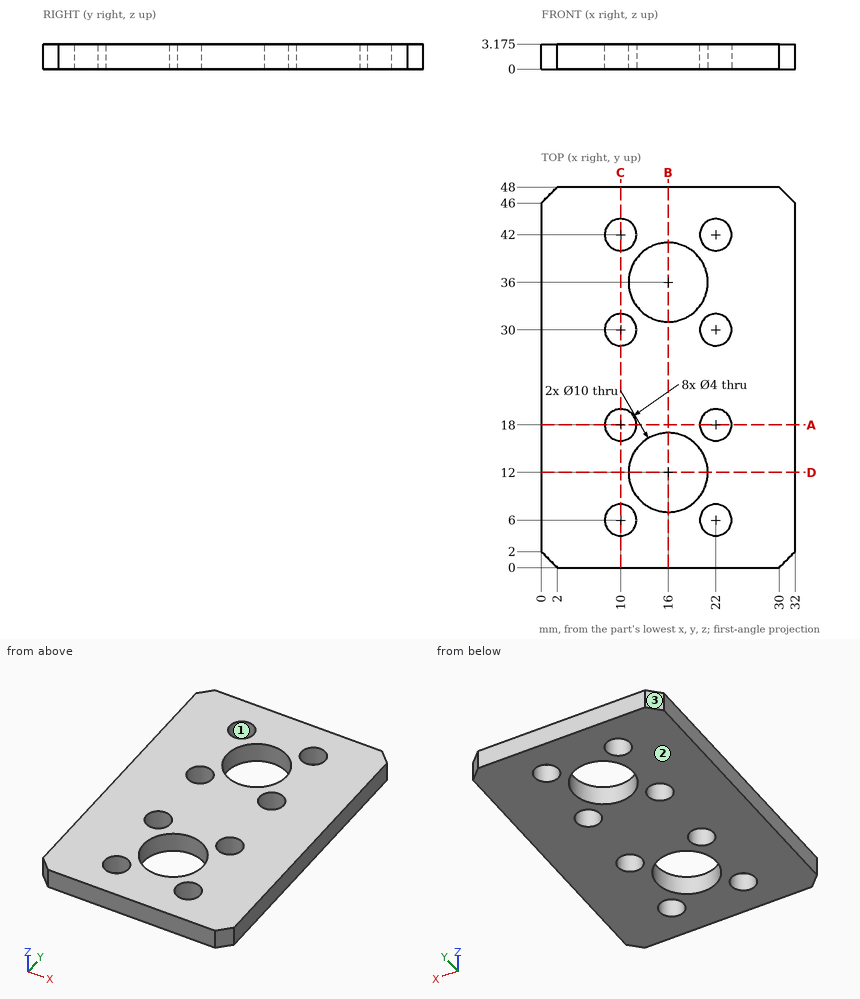
For this review, use the dimensioned drawing (mm, ordinates from the lowest corner) and the shaded views. Give positions to 0.01 mm unless a question says otherwise; leave off trailing zeros. Write each loop counter-clockwise with the first axis right and the second up, starting at its lowest first coordinate (ties: lowest second). Pieces come first, ordered by that corner, then holes. Notation, with made-up numbers: M 63,-9.75 L 98,-9.75 A11 cw 98,7.25 Z; hole C -8,22.5 d6. An arc over 180 degrees is marked long. Answer as a JSON object with one key per item and string values. Group by question number.
1) For line 1 along Y through (x, z) = (16, 0.75); line 2 along Y through (x, z) = (22, 1.75); line 3 along X through (y, z) = (39, 1.5), list the stretches that pass through material, from the lowest coordinate up.
2) We need section B-B (x = 16). Give the boundary of the cut face in (y, z) (3 decimals), and give its area (3 significant figures).
3) We need section A-A (y = 18). Give the boundary of the cut face in (x, z) (3 decimals).
4) We need section D-D (y = 12). Give the boundary of the cut face in (x, z) (3 decimals).
5) Mouldability with a two-part tool opening along X and no side actions: class the marked faces 1, 2 and 3 as released by +X, released by -X, zero draft, split by the parting line, or undercut.
6) We need section C-C (x = 10). Give the boundary of the cut face in (y, z) (3 decimals), and give its area (3 significant figures).
Answer key:
{
 "1": {"line 1": "y = 0 to 7, 17 to 31, 41 to 48", "line 2": "y = 0 to 4, 8 to 16, 20 to 28, 32 to 40, 44 to 48", "line 3": "x = 0 to 12, 20 to 32"},
 "2": {"outline": "M 0,0 L 7,0 L 7,3.175 L 0,3.175 Z; M 17,0 L 31,0 L 31,3.175 L 17,3.175 Z; M 41,0 L 48,0 L 48,3.175 L 41,3.175 Z", "area": "88.9 mm²"},
 "3": {"outline": "M 0,0 L 8,0 L 8,3.175 L 0,3.175 Z; M 12,0 L 20,0 L 20,3.175 L 12,3.175 Z; M 24,0 L 32,0 L 32,3.175 L 24,3.175 Z"},
 "4": {"outline": "M 0,0 L 11,0 L 11,3.175 L 0,3.175 Z; M 21,0 L 32,0 L 32,3.175 L 21,3.175 Z"},
 "5": {"face 1": "undercut", "face 2": "zero draft", "face 3": "released by -X"},
 "6": {"outline": "M 0,0 L 4,0 L 4,3.175 L 0,3.175 Z; M 8,0 L 16,0 L 16,3.175 L 8,3.175 Z; M 20,0 L 28,0 L 28,3.175 L 20,3.175 Z; M 32,0 L 40,0 L 40,3.175 L 32,3.175 Z; M 44,0 L 48,0 L 48,3.175 L 44,3.175 Z", "area": "102 mm²"}
}
